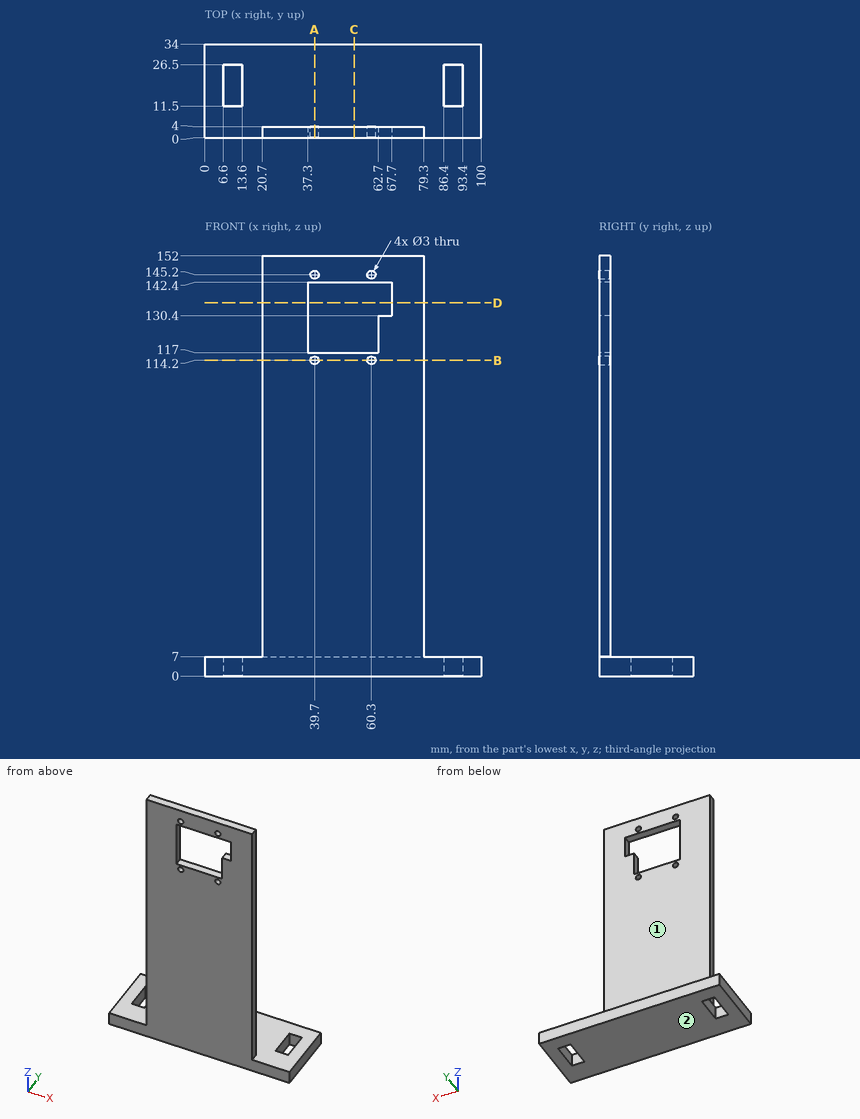
The drawing under review shows one solid part. Ordinate dimensions are in mm from its lowest x, y, z. A direction names the side the tool comes from. Round coordinates to 2 decimals unless told otherwise and drop trailing zeros. Loops run counter-clockwise (first coordinate to the right, second up) from the corner with the lowest first, then second, coordinate; pieces in that order, holes last. Notation, with made-up numbers: (30, -14) - (41, -14) arc R35 cw to (41, 19) - close; hole circle Ø3 at (44.5, 86). An arc over 180 degrees is marked (long way). One line per item, written item: value. Start each with the question number.
1) Consider section B-B on z = 114.2. Give the boundary of the cut face in (x, y).
2) To check wall thickness, follow L1, parallel to X at y = 1.95, z = 145.2; L2, parallel to Z at x = 60, y = 2; L3, parallel to Z at x = 18, y = 26.5. State the ranges of each line that lie inside material, in increasing order. Write a range as from..to.
3) Insertion check: pin 1 Ø12 at (x, z) = (18.5, 123.5) entering from +Y; pin 2 Ø7.5 at (y, z) = (17.5, 5) entering from -X; pin 3 Ø4.5 at (y, z) = (2, 103) entering from -X; pin 4 Ø10 at (x, y) = (59, 10) entering from +Z. Each pin has a flat end and moves straight along its axis. Give the tip position at first contact, or say it passes through.
4) For the marked faces 1 and 2, list the 3-axis set-ups (+Z, -Z, +X, -X, +Y, -Y) from which the entire face can be reached by the end or side of a thin tool; tool diameter is ignored.
5) Consider section D-D on z = 135. Give the boundary of the cut face in (x, y), then the cut area to 3 significant figures.
6) Consider section A-A on x = 39.7. Give the boundary of the cut face in (y, z).
7) Consider section C-C on x = 54. Give the boundary of the cut face in (y, z), then the cut area to 3 significant figures.
Reported:
1. outline: (20.7, 0) - (38.2, 0) - (38.2, 4) - (20.7, 4) - close; (41.2, 0) - (58.8, 0) - (58.8, 4) - (41.2, 4) - close; (61.8, 0) - (79.3, 0) - (79.3, 4) - (61.8, 4) - close
2. L1: x = 20.7..38.2, 41.2..58.8, 61.8..79.3
2. L2: z = 0..112.73, 115.67..117, 142.4..143.73, 146.67..152
2. L3: z = 0..7
3. pin 1: stops at y = 4
3. pin 2: stops at x = 0
3. pin 3: stops at x = 20.7
3. pin 4: stops at z = 7
4. face 1: +Z, +X, -X, +Y
4. face 2: -Z, +X, -X, +Y, -Y
5. outline: (20.7, 0) - (37.3, 0) - (37.3, 4) - (20.7, 4) - close; (67.7, 0) - (79.3, 0) - (79.3, 4) - (67.7, 4) - close
5. area: 113 mm^2
6. outline: (0, 0) - (34, 0) - (34, 7) - (4, 7) - (4, 112.7) - (0, 112.7) - close; (0, 115.7) - (4, 115.7) - (4, 117) - (0, 117) - close; (0, 142.4) - (4, 142.4) - (4, 143.7) - (0, 143.7) - close; (0, 146.7) - (4, 146.7) - (4, 152) - (0, 152) - close
7. outline: (0, 0) - (34, 0) - (34, 7) - (4, 7) - (4, 117) - (0, 117) - close; (0, 142.4) - (4, 142.4) - (4, 152) - (0, 152) - close
7. area: 716 mm^2
